from build123d import *

# Parameters (mm, degrees)
SKETCH1_W           = 46.85
SKETCH1_H           = 26.3
SKETCH1_W_2         = 26.3
SKETCH1_H_2         = 46.85
BOSS_EXTRUDE1_DEPTH = 5


with BuildPart() as part:
    # Sketch1 → Boss-Extrude1 (new body)
    with BuildSketch(Plane.XY):
        with Locations((-36.575, 0)):
            Rectangle(SKETCH1_W, SKETCH1_H)
        Rectangle(SKETCH1_W_2, SKETCH1_H)
        with Locations((36.575, 0)):
            Rectangle(SKETCH1_W, SKETCH1_H)
        with Locations((0, -36.575)):
            Rectangle(SKETCH1_W_2, SKETCH1_H_2)
        with Locations((0, 36.575)):
            Rectangle(SKETCH1_W_2, SKETCH1_H_2)
    extrude(amount=BOSS_EXTRUDE1_DEPTH)


solid = part.part
Source: CAD feature listing. Evaluate the final solid. Frame: model axes, mm. A direction names the side the tool comes from. Give positions to 0.01 mm unless a question says otherwise; leave off trailing zeros. Write each loop counter-clockwise with the first axis right and the second up, starting at its lowest first coordinate (ties: lowest second). Pieces come first, ordered by that corner, then holes. Notation, with made-up numbers: (35.25, 38) -> (62.25, 38) arc R9 cw to (62.25, 47) -> close; hole circle Ø9 at (34.5, 34.5). An arc over 180 degrees is marked (long way). Return JSON: item names as keys, results as strings. Group by question number.
1. Material intervals for line 1 (Y direction, x = -53, z = 2.3), sorted ascending. Write a range as from..to.
2. Section A-A, the plane z = 3.05. Output: boundary loops of the cut face in (x, y).
3. Section B-B, the plane y = -17. Output: boundary loops of the cut face in (x, z).
4. Access query for faces 1 (the face through (-13.15, -37, 2)), 2 (the face through (-36, 13.15, 2)), 3 (the face through (37, 13.15, 2)), 4 (the face through (13.15, -37, 2)). Directions: +Z, -Z, +X, -X, +Y, -Y. A direction counts if a zero-diameter tool reaches every point of the face in a straight line with its end or side. Return the directions, or none.
5. Pin query (flat end, axial travel): pin 1 Ø2.5 at (x, z) = (-27, 3.5) entering from +Y; pin 2 Ø2.5 at (y, z) = (-31, 3) entering from -X; pin 3 Ø1.5 at (y, z) = (38.5, 1.5) entering from +X. Return the tip coordinate at first contact, or that it passes through.
Determined:
{
 "1": {"line 1": "y = -13.15..13.15"},
 "2": {"outline": "(-60, -13.15) -> (-13.15, -13.15) -> (-13.15, -60) -> (13.15, -60) -> (13.15, -13.15) -> (60, -13.15) -> (60, 13.15) -> (13.15, 13.15) -> (13.15, 60) -> (-13.15, 60) -> (-13.15, 13.15) -> (-60, 13.15) -> close"},
 "3": {"outline": "(-13.15, 0) -> (13.15, 0) -> (13.15, 5) -> (-13.15, 5) -> close"},
 "4": {"face 1": "+Z, -Z, -X, -Y", "face 2": "+Z, -Z, -X, +Y", "face 3": "+Z, -Z, +X, +Y", "face 4": "+Z, -Z, +X, -Y"},
 "5": {"pin 1": "stops at y = 13.15", "pin 2": "stops at x = -13.15", "pin 3": "stops at x = 13.15"}
}
